Geometry: see drawing. Coordinates: mm, zero at the bounding-box minimum. A direction names the side the tool comes from. Coordinates: 2 decimals unless noted, no trailing zeros. Order: outer loops, then holes, each group sorted by start corner. A loop starts at its lowest first (then second) coordinate and runs counter-clockwise, first axis right, second up. Notation, with made-up numbers: (88.25, 81.5) -> (112.25, 81.5) arc R18 cw to (112.25, 90.5) -> close; hole circle Ø2 at (-13.75, 72). An arc over 180 degrees is marked (long way). One line per item, written item: value. Start each with the question number.
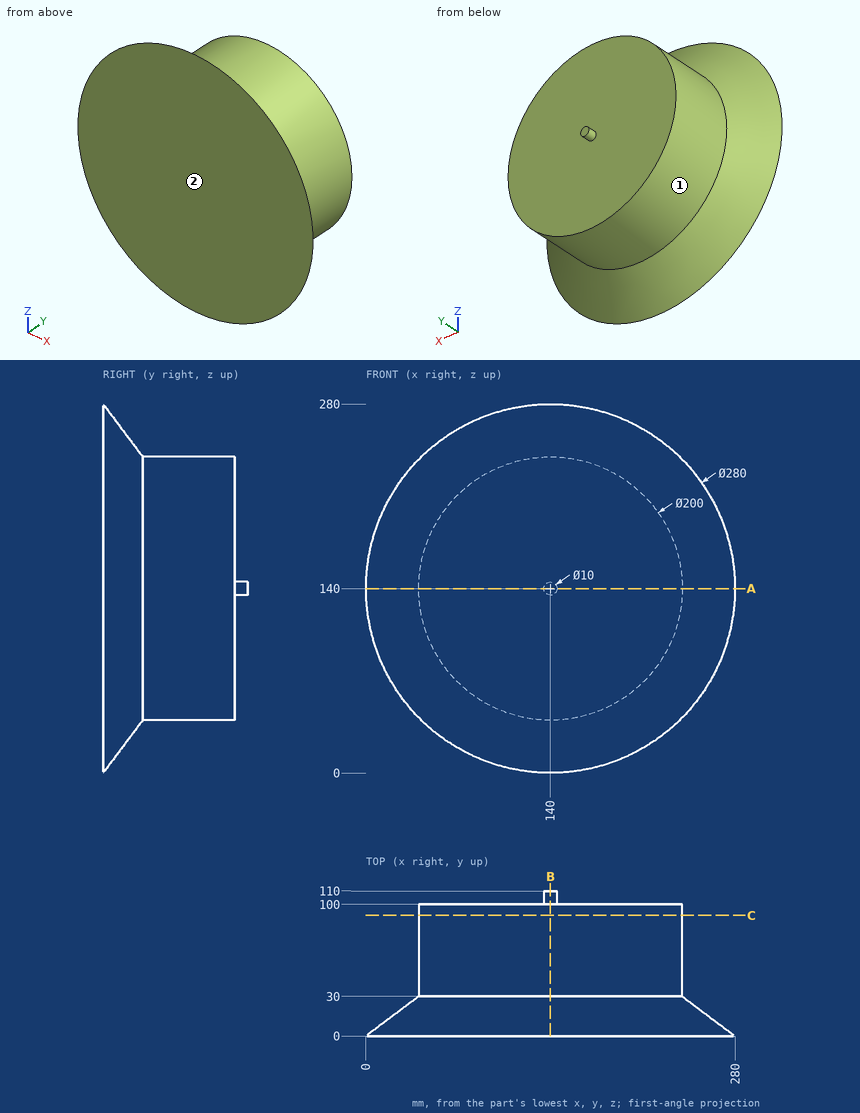
1) Section query A-A, the plane z = 140. Return the cut outline in (x, y).
2) Pin query (flat end, axial travel): pin 1 Ø3 at (y, z) = (11, 154) entering from -X; pin 2 Ø1.5 at (y, z) = (36, 157.5) entering from +X; pin 3 Ø5 at (x, z) = (91.5, 60) entering from -Y; pin 4 Ø2 at (x, y) = (89.5, 96) entering from -Z. Return the tip coordinate at first contact, or that it passes through.
3) Section query C-C, the plane y = 91.5. Return the cut outline in (x, z).
4) Section query B-B, the plane x = 140. Return the cut outline in (y, z), plus the area to 3 significant figures.
5) Ray query, line 1 along Y through (x, z) = (140.5, 220); line 2 along X through (y, z) = (43, 132.5); line 3 along X through (y, z) = (91.5, 104). Return the intervals inside material, ascending. Write a range as from..to.
6) Access query for the marked faces 1 and 2. Directions: +Z, -Z, +X, -X, +Y, -Y. A direction counts if a zero-diameter tool reaches every point of the face in a straight line with its end or side. Return the directions, or none.
Entries:
1. outline: (0, 0) -> (280, 0) -> (240, 30) -> (240, 100) -> (145, 100) -> (145, 110) -> (135, 110) -> (135, 100) -> (40, 100) -> (40, 30) -> close
2. pin 1: stops at x = 13.43
2. pin 2: stops at x = 238.59
2. pin 3: stops at y = 0
2. pin 4: stops at z = 53.11
3. outline: circle Ø200 at (140, 140)
4. outline: (0, 0) -> (30, 40) -> (100, 40) -> (100, 135) -> (110, 135) -> (110, 145) -> (100, 145) -> (100, 240) -> (30, 240) -> (0, 280) -> close
4. area: 21,300 mm2
5. line 1: y = 0..100
5. line 2: x = 40.28..239.72
5. line 3: x = 46.7..233.3
6. face 1: +Y
6. face 2: +Z, -Z, +X, -X, -Y
